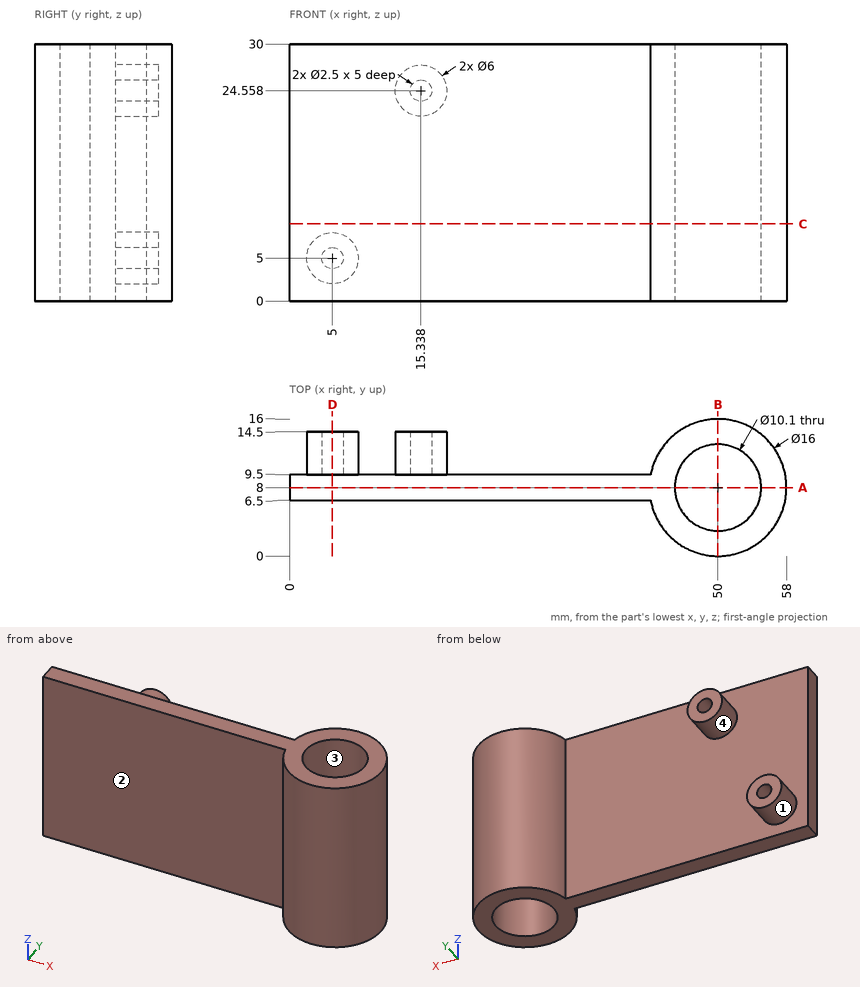
For this review, use the dimensioned drawing (mm, ordinates from the lowest corner) and the shaded views. A direction names the side the tool comes from. Coordinates: 2 decimals unless noted, no trailing zeros. Order: outer loops, then holes, each group sorted by start corner. A loop starts at its lowest first (then second) coordinate and runs counter-clockwise, first axis right, second up. Notation, with made-up numbers: (2.5, 47.25) - (54.5, 47.25) arc R18 cw to (54.5, 71.25) - close; hole circle Ø10 at (36.25, 69.25). An arc over 180 degrees is marked (long way). Answer as a JSON object with one key per item and string values. Group by question number.
1. We need section C-C on z = 9. State the section outline as (x, y) points.
2. We need section D-D on x = 5. State the section outline as (y, z) points, then the cut area to 4 significant figures.
3. For the marked faces 3 and 4, list the 3-axis set-ups (+Z, -Z, +X, -X, +Y, -Y) from which the entire face can be reached by the end or side of a thin tool; tool diameter is ignored.
4. We need section B-B on x = 50. State the section outline as (y, z) points.
5. We need section A-A on y = 8. State the section outline as (x, z) points.
6. Clearance check with flat-ended pins moving along their axes: P1, Ø4, axis at y = 3.5, z = 19, coming from the +X side; P2, Ø3, axis at x = 15.5, z = 25, coming from the +Y side; P3, Ø1.5, axis at x = 15.34, z = 24.56, coming from the +Y side; P4, Ø6, axis at x = 51.5, y = 3.5, coming from the +Z side. State where each tip first meets the part, or that it passes through.
7. For probe 1 along X at (y, z) = (12.15, 5); probe 2 along X at (y, z) = (11, 23.5) (1 decimal); probe 3 along Y at (x, z) = (7, 18), list the stretches that pass through material, from the lowest coordinate up.
8. The part is to be moulded in two halves that separate along X. For the marked faces 1 and 2, say which applies: pulls with the +X half, pulls with the -X half, needs draft (parallel to the pull), parting line crosses it, or undercut.
Final values:
{
 "1": {"outline": "(0, 6.5) - (42.14, 6.5) arc R8 ccw (long way) to (42.14, 9.5) - (0, 9.5) - close; hole circle Ø10.1 at (50, 8)"},
 "2": {"outline": "(6.5, 0) - (9.5, 0) - (9.5, 2) - (14.5, 2) - (14.5, 3.75) - (9.5, 3.75) - (9.5, 6.25) - (14.5, 6.25) - (14.5, 8) - (9.5, 8) - (9.5, 30) - (6.5, 30) - close", "area": "107.5 mm²"},
 "3": {"face 3": "+Z, -Z", "face 4": "+Y"},
 "4": {"outline": "(0, 0) - (2.95, 0) - (2.95, 30) - (0, 30) - close; (13.05, 0) - (16, 0) - (16, 30) - (13.05, 30) - close"},
 "5": {"outline": "(0, 0) - (44.95, 0) - (44.95, 30) - (0, 30) - close; (55.05, 0) - (58, 0) - (58, 30) - (55.05, 30) - close"},
 "6": {"P1": "x = 57.6", "P2": "y = 14.5", "P3": "y = 9.5", "P4": "z = 30"},
 "7": {"probe 1": "2 to 3.75, 6.25 to 8, 43.16 to 47.12, 52.88 to 56.84", "probe 2": "12.5 to 14.7, 16 to 18.1, 42.6 to 45.9, 54.1 to 57.4", "probe 3": "6.5 to 9.5"},
 "8": {"face 1": "undercut", "face 2": "needs draft"}
}
